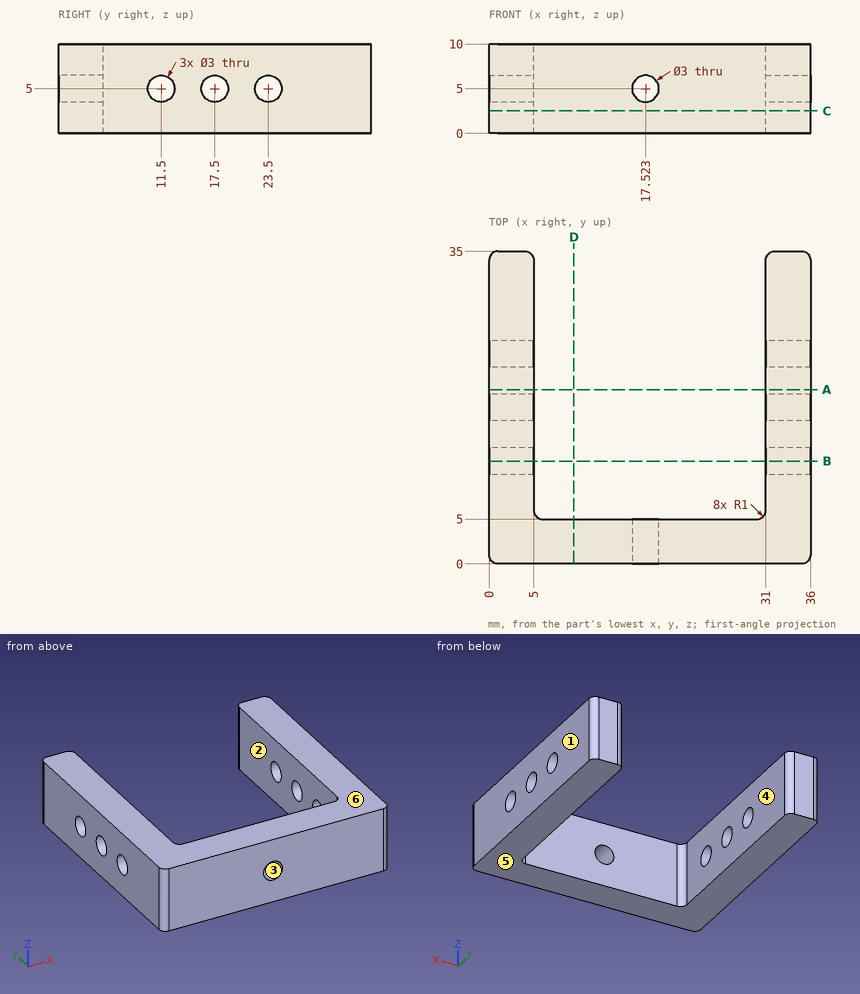
Part print with two shaded views. Sizes in mm from the minimum x, y, z corner. A direction names the side the tool comes from. Coordinates: 2 decimals unless noted, no trailing zeros. Write each loop counter-clockwise with the first axis right and the second up, starting at its lowest first coordinate (ties: lowest second). Pieces come first, ordered by that corner, then holes. Notation, with made-up numbers: (70, 53.25) - (113, 53.25) arc R27 cw to (113, 78.25) - close; hole circle Ø11 at (87, -38). An arc over 180 degrees is marked (long way). Use a Markdown table: item, result. Add a question column.
Item 1: Two-plate mould, pull along Z, no slides. Class the marked faces 3, 4, 5 and 6: pulls with the +Z half, pulls with the -Z half, needs draft (parallel to the pull), parting line crosses it, or undercut.
Item 2: 3-axis set-ups, long thin cutter, end or side, ignore diameter. For the marked faces 1 and 2: which of +Z, -Z, +X, -X, +Y, -Y reach the whole face in a straight line?
Item 3: Band-saw the part on D-D, the plane x = 9.5. Write the cut outline in (y, z).
Item 4: Band-saw the part on C-C, the plane z = 2.5. Write the cut outline in (x, y).
Item 5: Drop a flat-ended pin along its axis: pin 1 (3 mm diameter, centred on x = 16.5, z = 2.5, fed in from +Y). Give the stop position or say it passes through.
Item 6: Band-saw the part on B-B, the plane y = 11.5. Write the cut outline in (x, z), and give its area (3 significant figures).
Item 7: Drill centre lines: line 1 along Y through (x, z) = (32.2, 5); line 2 along X through (y, z) = (21.5, 8.75); line 3 along Y through (x, z) = (26, 1.25). Where is each one in solid material? Low to high.
Item 8: Band-saw the part on A-A, the plane y = 19.5. Write the cut outline in (x, z), and give its area (3 significant figures).
A:
| question | item | result |
|---|---|---|
| 1 | face 3 | undercut |
| 1 | face 4 | needs draft |
| 1 | face 5 | pulls with the -Z half |
| 1 | face 6 | pulls with the +Z half |
| 2 | face 1 | +Z, -Z, +X, +Y, -Y |
| 2 | face 2 | +Z, -Z, +Y |
| 3 | outline | (0, 0) - (5, 0) - (5, 10) - (0, 10) - close |
| 4 | outline | (0, 1) arc R1 ccw to (1, 0) - (35, 0) arc R1 ccw to (36, 1) - (36, 34) arc R1 ccw to (35, 35) - (32, 35) arc R1 ccw to (31, 34) - (31, 6) arc R1 cw to (30, 5) - (6, 5) arc R1 cw to (5, 6) - (5, 34) arc R1 ccw to (4, 35) - (1, 35) arc R1 ccw to (0, 34) - close |
| 5 | pin 1 | stops at y = 5 |
| 6 | outline | (0, 0) - (5, 0) - (5, 3.5) - (0, 3.5) - close; (0, 6.5) - (5, 6.5) - (5, 10) - (0, 10) - close; (31, 0) - (36, 0) - (36, 3.5) - (31, 3.5) - close; (31, 6.5) - (36, 6.5) - (36, 10) - (31, 10) - close |
| 6 | area | 70.0 mm² |
| 7 | line 1 | y = 0 to 10, 13 to 16, 19 to 22, 25 to 35 |
| 7 | line 2 | x = 0 to 5, 31 to 36 |
| 7 | line 3 | y = 0 to 5 |
| 8 | outline | (0, 0) - (5, 0) - (5, 10) - (0, 10) - close; (31, 0) - (36, 0) - (36, 10) - (31, 10) - close |
| 8 | area | 100 mm² |
